Could you check a few things on this model? Use its own coordinates, in mm. Give positions to 0.01 mm unless a question says otherwise; leave off trailing zeros. Loops run counter-clockwise (first coordinate to the right, second up) from the corner with the lowest first, then second, coordinate; pieces in that order, holes last. Notation, with made-up numbers: M 74.25,12 L 89.25,12 A18 cw 89.25,43 Z; hole C 8.25,51 d5. An arc over 180 degrees is marked long. Return JSON: item names as keys, results as strings. Group by question number.
1. For pin 1 (2 mm diameter, centred on y = -4, z = 14.5, fed in from +X); pin 2 (2 mm diameter, centred on y = 1, z = -1, fed in from -X); pin 3 (8 mm diameter, centred on x = -9, y = -5.5, fed in from -Z); pin 4 (1.5 mm diameter, centred on x = -17.5, y = -14, fed in from +Z), each with a flat end and sliding along its axis, tell me the tip position at first contact or that it passes through.
2. If we section it at D-D (y = -16): Write out the boundary of the cut face in (x, z).
3. If we mould it in two halves opening along Y, with no side actions, what happens to faces 1 (the cylindrical face through (-23.259, 10.906, 1.432)), 2 (the flat face through (-30, -5, 0)), 3 (the flat face through (-27, 3.5, 0))? For each: +Y half, -Y half, draft (parallel to the pull), parting line (faces both ways), or undercut.
4. If we section it at A-A (y = 0): Write out the boundary of the cut face in (x, z).
5. Please list where these lines run through material, in increasing order: line 1 (Z direction, x = -6.5, y = -3); line 2 (Z direction, x = -12.5, y = 5.5); line 3 (X direction, y = 7.5, z = -17).
6. If we section it at C-C (x = -21): Write out the boundary of the cut face in (y, z), plus the area to 3 significant figures.
```python
from build123d import *

# Parameters (mm, degrees)
SKETCH3_R           = 11
BOSS_EXTRUDE1_DEPTH = 30
SKETCH4_W           = 7
SKETCH4_H           = 7
CUT_EXTRUDE1_DEPTH  = 6


with BuildPart() as part:
    # Sketch1 → Revolve1 (revolve)
    with BuildSketch(Plane.XY):
        with BuildLine():
            Line((20, 0), (-20, 0))
            ThreePointArc((-20, 0), (0, 20), (20, 0))
        make_face()
    revolve(axis=Axis((-20, 0, 0), (1, 0, 0)))

    # Sketch3 → Boss-Extrude1 (add)
    with BuildSketch(Plane(origin=(0, 0, 0), x_dir=(0, 0, -1), z_dir=(1, 0, 0))):
        Circle(SKETCH3_R)
    extrude(amount=-BOSS_EXTRUDE1_DEPTH)

    # Sketch4 → Cut-Extrude1 (cut)
    with BuildSketch(Plane.ZY.offset(30)):
        Rectangle(SKETCH4_W, SKETCH4_H)
    extrude(amount=-CUT_EXTRUDE1_DEPTH, mode=Mode.SUBTRACT)


solid = part.part
```
Answer:
{
 "1": {"pin 1": "stops at x = 14.24", "pin 2": "stops at x = -24", "pin 3": "stops at z = -18.9", "pin 4": "passes through"},
 "2": {"outline": "C 0,0 d24"},
 "3": {"face 1": "parting line", "face 2": "draft", "face 3": "undercut"},
 "4": {"outline": "M -30,-11 L -16.7,-11 A20 ccw long -16.7,11 L -30,11 L -30,3.5 L -24,3.5 L -24,-3.5 L -30,-3.5 Z"},
 "5": {"line 1": "z = -18.67 to 18.67", "line 2": "z = -14.61 to 14.61", "line 3": "x = -7.4 to 7.4"},
 "6": {"outline": "C 0,0 d22", "area": "380 mm²"}
}
